```python
from build123d import *

# Parameters (mm, degrees)
F0_W     = 130
F0_H     = 60
F0_R     = 2.55
F0_W_2   = 7
F0_H_2   = 15
F1_DEPTH = 3
F2_R     = 5


with BuildPart() as f1:
    # F0 (on Top) → F1 (new body)
    with BuildSketch(Plane.XY):
        with Locations((65, 30)):
            Rectangle(F0_W, F0_H)
        with Locations((6, 6)):
            Circle(F0_R, mode=Mode.SUBTRACT)
        with Locations((124, 6)):
            Circle(F0_R, mode=Mode.SUBTRACT)
        with Locations((18.5, 30)):
            Rectangle(F0_W_2, F0_H_2, mode=Mode.SUBTRACT)
        with Locations((6, 54)):
            Circle(F0_R, mode=Mode.SUBTRACT)
        with Locations((111.5, 30)):
            Rectangle(F0_W_2, F0_H_2, mode=Mode.SUBTRACT)
        with Locations((124, 54)):
            Circle(F0_R, mode=Mode.SUBTRACT)
    extrude(amount=F1_DEPTH)

    # F2
    f2_edges = [f1.edges().sort_by_distance(p)[0] for p in [
        (130, 0, 1.5),
        (130, 60, 1.5),
        (0, 0, 1.5),
        (0, 60, 1.5),
    ]]
    fillet(f2_edges, radius=F2_R)


solid = f1.part
```
Here's how the part is built. I have some questions about the finished solid (model axes, mm). A direction names the side the tool comes from. Coordinates: 2 decimals unless noted, no trailing zeros. Order: outer loops, then holes, each group sorted by start corner. A loop starts at its lowest first (then second) coordinate and runs counter-clockwise, first axis right, second up. Notation, with made-up numbers: M 71,-34.5 L 128,-34.5 A21 ccw 128,-0.5 Z; hole C 27.5,55 d3. An arc over 180 degrees is marked long. Answer as a JSON object with one key per item and string values. Group by question number.
(1) Suppose I cut it at A-A, the plane z = 1. Please give me the cut outline in (x, y), then the cut area to 3 significant figures.
(2) I need wall thicknesses on probe 1 along Y at (x, z) = (6, 0.7); probe 2 along X at (y, z) = (29, 1.45); probe 3 along X at (y, z) = (52, 2.8). Which ranges of each line are inside material? Lowest first, please.
(3) If we mould it in two halves opening along X, with no side actions, what happens to faces 1 (the face through (126.43, 54.77, 1.48)), 2 (the face through (128, 1, 2)), 3 (the face through (1, 2, 2))? For each: released by +X, released by -X, zero draft, split by the parting line, or undercut.
(4) Which directions (+Z, -Z, +X, -X, +Y, -Y) give clear straight access to the entire face, cutting with the end or side of a thin tool? Please do faces 4 (the face through (128, 59, 2)), 5 (the face through (15, 30, 1)).
Values found:
{
 "1": {"outline": "M 0,5 A5 ccw 5,0 L 125,0 A5 ccw 130,5 L 130,55 A5 ccw 125,60 L 5,60 A5 ccw 0,55 Z; hole C 6,6 d5.1; hole C 6,54 d5.1; hole M 15,22.5 L 22,22.5 L 22,37.5 L 15,37.5 Z; hole M 108,22.5 L 115,22.5 L 115,37.5 L 108,37.5 Z; hole C 124,6 d5.1; hole C 124,54 d5.1", "area": "7,490 mm^2"},
 "2": {"probe 1": "y = 0 to 3.45, 8.55 to 51.45, 56.55 to 60", "probe 2": "x = 0 to 15, 22 to 108, 115 to 130", "probe 3": "x = 0 to 4.42, 7.58 to 122.42, 125.58 to 130"},
 "3": {"face 1": "undercut", "face 2": "released by +X", "face 3": "released by -X"},
 "4": {"face 4": "+Z, -Z, +X, +Y", "face 5": "+Z, -Z"}
}
